Geometry: final body of the model. Coordinates: model frame, mm. Coordinates: 2 decimals unless noted, no trailing zeros. Order: outer loops, then holes, each group sorted by start corner. A loop starts at its lowest first (then second) coordinate and runs counter-clockwise, first axis right, second up. Notation, with made-up numbers: (30, 1.5) - (86, 1.5) arc R19 cw to (86, 24.5) - close; hole circle Ø10 at (59.5, 71.25). An arc over 180 degrees is marked (long way). Use a Markdown table: item, result. Add a question column.
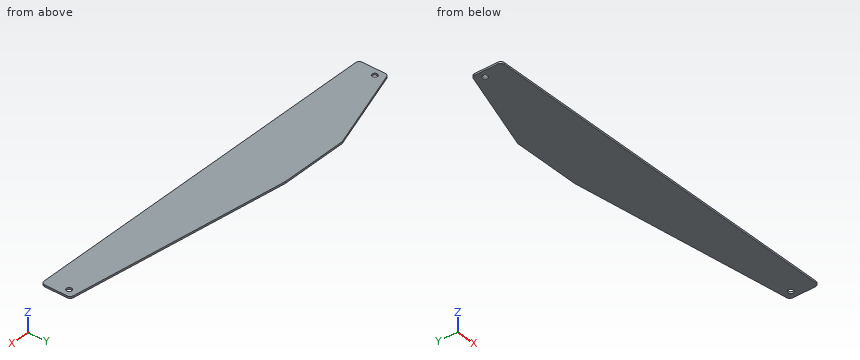
Autodesk Inventor part; units mm, degrees
ref_plane "YZ Plane" through (0, 0, 0) normal (1, 0, 0) x (0, 1, 0)
ref_plane "XZ Plane" through (0, 0, 0) normal (0, 1, 0) x (-1, 0, 0)
ref_plane "XY Plane" through (0, 0, 0) normal (0, 0, 1) x (1, 0, 0)
sketch "Sketch1" plane through (0, 0, 0) normal (0, 0, 1) x (1, 0, 0)
  circle A0 centre (-120.15, 28.2703) radius 2.3114
  circle A1 centre (-437.65, 28.2703) radius 2.3114
  line L0 (-124.0119, 9.2203) -> (-113.8, 9.2203)
  line L1 (-113.8, 24.2317) -> (-113.8, 32.2073)
  line L2 (-443.67, 33.8077) -> (-443.67, 0.5333)
  line L3 (-382.9881, 34.6203) -> (-441.5119, 34.6203)
  line L4 (-443.67, 34.6203) -> (-113.8, 34.6203)
  line L5 (-113.8, 31.8362) -> (-113.8, 12.3953)
  line L6 (-116.975, 9.2203) -> (-440.495, 9.2203)
  line L7 (-443.67, 12.3953) -> (-443.67, 32.316)
  arc A2 (-116.975, 9.2203) -> (-113.8, 12.3953) centre (-116.975, 12.3953) ccw
  circle A3 centre (-361.45, 54.8387) radius 2.3114
  line L8 (-306.586, 60.0203) -> (-365.773, 60.0203)
  line L9 (-365.773, 60.0203) -> (-441.4793, 35.3346)
  line L10 (-306.586, 60.0203) -> (-116.5603, 34.984)
  arc A4 (-443.67, 12.3953) -> (-440.495, 9.2203) centre (-440.495, 12.3953) ccw
  arc A5 (-441.4793, 35.3346) -> (-443.67, 32.316) centre (-440.495, 32.316) ccw
  arc A6 (-113.8, 31.8362) -> (-116.5603, 34.984) centre (-116.975, 31.8362) ccw
  line L11 (-306.586, 60.0203) -> (-365.773, 60.0203)
  point P0 (0, 0)
  dimension "d0" = 3.175
  dimension "d1" = 3.175
extrude "Extrusion1" add sketch "Sketch1" along normal blind 1.5875
sketch "Sketch2" plane through (0, 0, 1.5875) normal (0, 0, 1) x (1, 0, 0)
  circle A0 centre (-361.45, 54.8387) radius 2.3114
  circle A1 centre (-361.45, 54.8387) radius 2.3114
  point P0 (0, 0)
extrude "Extrusion2" add sketch "Sketch2" against normal blind 1.5875
properties part number "panel"
1) Line query: line 1 (Y direction, x = -120.15, z = 1.2); line 2 (Y direction, x = -437.65, z = 0.7); line 3 (X direction, y = 12, z = 0.55). Output: solid intervals per line, ascending. Write a range as from..to.
2) First-contact query: pin 1 (4 mm diameter, centred on x = -120.15, y = 28.27, fed in from -Z). Flat tip, straight axial feed; report the tip coordinate or a pass-through.
3) Section query C-C (y = 38.5). Return the cut outline in (x, z), and give its area (3 significant figures).
4) Section query A-A (z = 0.25). Return the cut outline in (x, y) (3 decimals).
5) Section query B-B (x = -270). Return the cut outline in (y, z), and give its area (3 significant figures).
From the geometry:
| question | item | result |
|---|---|---|
| 1 | line 1 | y = 9.22..25.96, 30.58..35.46 |
| 1 | line 2 | y = 9.22..25.96, 30.58..36.58 |
| 1 | line 3 | x = -443.65..-113.82 |
| 2 | pin 1 | passes through |
| 3 | outline | (-431.77, 0) - (-143.25, 0) - (-143.25, 1.59) - (-431.77, 1.59) - close |
| 3 | area | 458 mm^2 |
| 4 | outline | (-443.67, 12.395) arc R3.175 ccw to (-440.495, 9.22) - (-116.975, 9.22) arc R3.175 ccw to (-113.8, 12.395) - (-113.8, 31.836) arc R3.175 ccw to (-116.56, 34.984) - (-306.586, 60.02) - (-365.773, 60.02) - (-441.479, 35.335) arc R3.175 ccw to (-443.67, 32.316) - close; hole circle Ø4.623 at (-437.65, 28.27); hole circle Ø4.623 at (-120.15, 28.27) |
| 5 | outline | (9.22, 0) - (55.2, 0) - (55.2, 1.59) - (9.22, 1.59) - close |
| 5 | area | 73.0 mm^2 |
